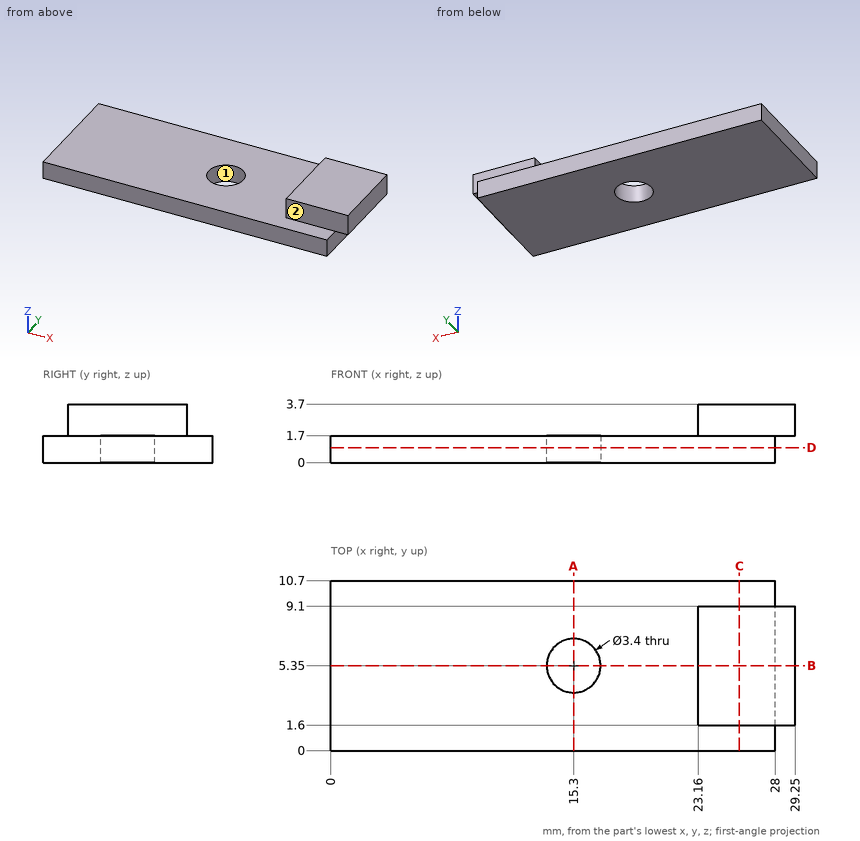
Verification items for this drawing (mm, ordinates from the low corner). Coordinates: 2 decimals unless noted, no trailing zeros. Write each loop counter-clockwise with the first axis right and the second up, starting at its lowest first coordinate (ties: lowest second). Pieces come first, ordered by that corner, then holes. Notation, with made-up numbers: M 35.5,67.25 L 39.5,67.25 A25 cw 39.5,85.25 Z; hole C 45,39 d9. An arc over 180 degrees is marked long. One line per item, written item: value. Start each with the question number.
(1) Sectioned sample at A-A, the plane x = 15.3. Enter the section's corners in (y, z), and give its area (3 significant figures).
(2) Scan lines: line 1 along Y through (x, z) = (15.3, 1.3); line 2 along Z through (x, y) = (28.25, 5.25); line 3 along X through (y, z) = (3.75, 2). Record each from-to range of solid material in increasing order. Write a range as [from, to].
(3) Sectioned sample at D-D, the plane z = 0.95. Enter the section's corners in (x, y).
(4) Release check for a two-part mould opening along X. For the marked faces 1 and 2 record: released by +X, released by -X, zero draft, split by the parting line, or undercut.
(5) Depth check by flat-ended pin: pin 1 (1.6 mm diameter, centred on x = 26.5, z = 3, fed in from -Y); pin 2 (1.9 mm diameter, centred on y = 6, z = 0.5, fed in from +X); pin 3 (2 mm diameter, centred on x = 25.5, z = 3, fed in from +Y). Enter the tip coordinate at first touch or a pass-through.
(6) Sectioned sample at B-B, the plane y = 5.35. Enter the section's corners in (x, z), and give its area (3 significant figures).
(7) Sectioned sample at C-C, the plane x = 25.75. Enter the section's corners in (y, z), and give its area (3 significant figures).
Filled sheet:
1. outline: M 0,0 L 3.65,0 L 3.65,1.7 L 0,1.7 Z; M 7.05,0 L 10.7,0 L 10.7,1.7 L 7.05,1.7 Z
1. area: 12.4 mm²
2. line 1: [0, 3.65], [7.05, 10.7]
2. line 2: [1.7, 3.7]
2. line 3: [23.16, 29.25]
3. outline: M 0,0 L 28,0 L 28,10.7 L 0,10.7 Z; hole C 15.3,5.35 d3.4
4. face 1: undercut
4. face 2: zero draft
5. pin 1: y = 1.6
5. pin 2: x = 28
5. pin 3: y = 9.1
6. outline: M 0,0 L 13.6,0 L 13.6,1.7 L 0,1.7 Z; M 17,0 L 28,0 L 28,1.7 L 29.25,1.7 L 29.25,3.7 L 23.16,3.7 L 23.16,1.7 L 17,1.7 Z
6. area: 54.0 mm²
7. outline: M 0,0 L 10.7,0 L 10.7,1.7 L 9.1,1.7 L 9.1,3.7 L 1.6,3.7 L 1.6,1.7 L 0,1.7 Z
7. area: 33.2 mm²
